Read the model definition and answer for the solid it produces. Units are mm, in the model's axes. A direction names the side the tool comes from. Round coordinates to 2 decimals unless told otherwise and drop trailing zeros. Write each loop counter-clockwise with the first axis right and the second up, starting at its lowest first coordinate (ties: lowest second). Pieces come first, ordered by that corner, then holes.
from build123d import *

# Parameters (mm, degrees)
SKETCH1_W                  = 63
SKETCH1_H                  = 118
BOSS_EXTRUDE1_DEPTH        = 35.5
SKETCH2_W                  = 60
SKETCH2_H                  = 115
CUT_EXTRUDE1_DEPTH         = 34
SKETCH3_W                  = 12.4
SKETCH3_H                  = 30.8
BOSS_EXTRUDE2_DEPTH        = 21.78
CUT_EXTRUDE2_REACH         = 129.081
SKETCH4_W                  = 10
SKETCH4_H                  = 27.8
CUT_EXTRUDE3_REACH         = 138.738
SKETCH5_W                  = 22.87
SKETCH5_H                  = 12.89
CUT_EXTRUDE4_REACH         = 138.738
SKETCH6_W                  = 22.87
SKETCH6_H                  = 12.89
CUT_EXTRUDE5_DEPTH         = 137.435882377
M2_5_CLEARANCE_HOLE1_D     = 3.05
M2_5_CLEARANCE_HOLE1_DEPTH = 35.5
M3_CLEARANCE_HOLE1_D       = 3.2512
M3_CLEARANCE_HOLE1_DEPTH   = 1.5
M3_CLEARANCE_HOLE2_D       = 3.2512
M3_CLEARANCE_HOLE2_DEPTH   = 63


with BuildPart() as part:
    # Sketch1 → Boss-Extrude1 (new body)
    with BuildSketch(Plane.XY.offset(34)):
        with Locations((30, 57.5)):
            Rectangle(SKETCH1_W, SKETCH1_H)
    extrude(amount=-BOSS_EXTRUDE1_DEPTH)

    # Sketch2 → Cut-Extrude1 (cut)
    with BuildSketch(Plane.XY.offset(34)):
        with Locations((30, 57.5)):
            Rectangle(SKETCH2_W, SKETCH2_H)
    extrude(amount=-CUT_EXTRUDE1_DEPTH, mode=Mode.SUBTRACT)

    # Sketch3 → Boss-Extrude2 (add)
    with BuildSketch(Plane.XY):
        with Locations((30, 27.9)):
            Rectangle(SKETCH3_W, SKETCH3_H)
    extrude(amount=BOSS_EXTRUDE2_DEPTH)

    # Sketch4 → Cut-Extrude2 (cut, up to next)
    with BuildSketch(Plane.ZY.offset(-23.8), mode=Mode.PRIVATE) as cut_extrude2_sk1:
        with Locations((16.78, 27.9)):
            Rectangle(SKETCH4_W, SKETCH4_H)
    cut_extrude2_tool1 = extrude(cut_extrude2_sk1.sketch, amount=-CUT_EXTRUDE2_REACH, mode=Mode.PRIVATE) & part.part
    add(cut_extrude2_tool1.solids().sort_by_distance((23.8, 27.9, 16.78))[0], mode=Mode.SUBTRACT)

    # Sketch5 → Cut-Extrude3 (cut, up to next)
    with BuildSketch(Plane(origin=(61.5, 0, 0), x_dir=(0, 0, -1), z_dir=(1, 0, 0)), mode=Mode.PRIVATE) as cut_extrude3_sk1:
        with Locations((-22.565, 16.805)):
            Rectangle(SKETCH5_W, SKETCH5_H)
    cut_extrude3_tool1 = extrude(cut_extrude3_sk1.sketch, amount=-CUT_EXTRUDE3_REACH, mode=Mode.PRIVATE) & part.part
    add(cut_extrude3_tool1.solids().sort_by_distance((61.5, 16.805, 22.565))[0], mode=Mode.SUBTRACT)

    # Sketch6 → Cut-Extrude4 (cut, up to next)
    with BuildSketch(Plane.ZY.offset(1.5), mode=Mode.PRIVATE) as cut_extrude4_sk1:
        with Locations((22.565, 16.805)):
            Rectangle(SKETCH6_W, SKETCH6_H)
    cut_extrude4_tool1 = extrude(cut_extrude4_sk1.sketch, amount=-CUT_EXTRUDE4_REACH, mode=Mode.PRIVATE) & part.part
    add(cut_extrude4_tool1.solids().sort_by_distance((-1.5, 16.805, 22.565))[0], mode=Mode.SUBTRACT)

    # Sketch7 → Cut-Extrude5 (cut, through all)
    with BuildSketch(Plane(origin=(0, 0, -1.5), x_dir=(-1, 0, 0), z_dir=(0, 0, -1))):
        with BuildLine():
            Line((-40, 55), (-20, 55))
            ThreePointArc((-20, 55), (-15, 60), (-20, 65))
            Line((-20, 65), (-40, 65))
            ThreePointArc((-40, 65), (-45, 60), (-40, 55))
        make_face()
    extrude(amount=-CUT_EXTRUDE5_DEPTH, mode=Mode.SUBTRACT)

    # M2.5 Clearance Hole1
    with Locations(Plane(origin=(0, 0, -1.5), x_dir=(-1, 0, 0), z_dir=(0, 0, -1))):
        with Locations((-9.95, 28.42), (-9.95, 21.935), (-50.05, 28.42), (-50.05, 21.935)):
            Hole(M2_5_CLEARANCE_HOLE1_D / 2, depth=M2_5_CLEARANCE_HOLE1_DEPTH)

    # M3 Clearance Hole1
    with Locations(Plane(origin=(0, 0, 0), x_dir=(0, 0, -1), z_dir=(1, 0, 0))):
        with Locations((-8.5, 57.5)):
            Hole(M3_CLEARANCE_HOLE1_D / 2, depth=M3_CLEARANCE_HOLE1_DEPTH)

    # M3 Clearance Hole2
    with Locations(Plane(origin=(61.5, 0, 0), x_dir=(0, 0, -1), z_dir=(1, 0, 0))):
        with Locations((-8.5, 57.5)):
            Hole(M3_CLEARANCE_HOLE2_D / 2, depth=M3_CLEARANCE_HOLE2_DEPTH)


solid = part.part
Q1. Determine the mould class of faces 6 (the flat face through (36.2, 28, 6)), 7 (the flat face through (0, 57, 17)), 8 (the flat face through (-0.5, 70.1, 34)), 9 (the flat face through (30, 116.5, 16)) for opening direction Y: pulls with the +Y half, pulls with the -Y half, needs draft (parallel to the pull), parting line crosses it, or undercut.
Verdict:
face 6: undercut
face 7: undercut
face 8: needs draft
face 9: pulls with the +Y half
Q2. A flat-ended cylindrical pin translates along its axis: pin 1 Ø0.8 at (x, y) = (28.5, 13.5) entering from +Z. Find the tip coordinate at first contact, or state that the pin passes through.
Verdict:
pin 1: stops at z = 21.78
Q3. Straight lines are drawn through the part: probe 1 along Y at (x, z) = (50.05, -0.5) (3 decimals); probe 2 along Y at (x, z) = (28, 20); probe 3 along X at (y, z) = (14.5, 1.5). For each, find the intervals that lie inside material, in ascending order.
Verdict:
probe 1: y = -1.5 to 20.41, 23.46 to 26.895, 29.945 to 116.5
probe 2: y = -1.5 to 0, 12.5 to 14, 41.8 to 43.3, 115 to 116.5
probe 3: x = -1.5 to 0, 23.8 to 36.2, 60 to 61.5
Q4. Section B-B (x = 9.95) is taken. Determine the outline of the cut face in (y, z) (3 decimals).
Verdict:
outline: (-1.5, -1.5) - (20.41, -1.5) - (20.41, 0) - (0, 0) - (0, 34) - (-1.5, 34) - close; (23.46, -1.5) - (26.895, -1.5) - (26.895, 0) - (23.46, 0) - close; (29.945, -1.5) - (116.5, -1.5) - (116.5, 34) - (115, 34) - (115, 0) - (29.945, 0) - close
Q5. Which of the six approach directions +Z, -Z, +X, -X, +Y, -Y give full straight-line access (tool end or side, diameter ignored) to faces 1 (the flat face through (61.5, 57, 16)), 2 (the flat face through (30, -1.5, 16)), 3 (the flat face through (30, 14, 17)), 4 (the flat face through (30, 41.8, 17)), 5 (the cylindrical face through (15, 60, -1))?
Verdict:
face 1: +Z, -Z, +X, +Y, -Y
face 2: +Z, -Z, +X, -X, -Y
face 3: +Z, +X, -X
face 4: +Z
face 5: +Z, -Z
Q6. Section C-C (z = 8.5) is taken. Determine the outline of the cut face in (x, y), then the cut area to 3 significant figures.
Verdict:
outline: (-1.5, -1.5) - (61.5, -1.5) - (61.5, 55.87) - (60, 55.87) - (60, 0) - (0, 0) - (0, 55.87) - (-1.5, 55.87) - close; (-1.5, 59.13) - (0, 59.13) - (0, 115) - (60, 115) - (60, 59.13) - (61.5, 59.13) - (61.5, 116.5) - (-1.5, 116.5) - close; (23.8, 12.5) - (36.2, 12.5) - (36.2, 43.3) - (23.8, 43.3) - close
area: 906 mm2
Q7. Section A-A (y = 28.42) is taken. Determine the outline of the cut face in (x, z) (3 decimals), then the cut area to 3 significant figures.
Verdict:
outline: (-1.5, -1.5) - (8.425, -1.5) - (8.425, 0) - (0, 0) - (0, 34) - (-1.5, 34) - close; (11.475, -1.5) - (48.525, -1.5) - (48.525, 0) - (36.2, 0) - (36.2, 11.78) - (23.8, 11.78) - (23.8, 0) - (11.475, 0) - close; (51.575, -1.5) - (61.5, -1.5) - (61.5, 34) - (60, 34) - (60, 0) - (51.575, 0) - close
area: 333 mm2
Q8. Section D-D (z = 32) is taken. Determine the outline of the cut face in (x, y).
Verdict:
outline: (-1.5, -1.5) - (61.5, -1.5) - (61.5, 10.36) - (60, 10.36) - (60, 0) - (0, 0) - (0, 10.36) - (-1.5, 10.36) - close; (-1.5, 23.25) - (0, 23.25) - (0, 115) - (60, 115) - (60, 23.25) - (61.5, 23.25) - (61.5, 116.5) - (-1.5, 116.5) - close
